Read the model definition and answer for the solid it produces. Units are mm, in the model's axes. A direction names the side the tool comes from. Give positions to 0.01 mm unless a question says otherwise; leave off trailing zeros. Write each loop counter-clockwise with the first axis right and the second up, starting at its lowest first coordinate (ties: lowest second). Pieces come first, ordered by that corner, then holes. Notation, with made-up numbers: (82, 44) -> (98, 44) arc R21 ccw to (98, 63) -> close; hole circle Ø7 at (10.5, 58). An arc over 180 degrees is marked (long way). Use a Markdown table: item, result.
from build123d import *

# Parameters (mm, degrees)
SKETCH1_W               = 325
SKETCH1_H               = 80
BOSS_EXTRUDE1_DEPTH     = 5
BOSS_EXTRUDE2_DEPTH     = 105
SKETCH3_R               = 4.5
CUT_EXTRUDE1_DEPTH      = 1
CUT_EXTRUDE1_DEPTH_BACK = 81
SKETCH4_W               = 120
SKETCH4_H               = 70
CUT_EXTRUDE2_DEPTH      = 105
SKETCH5_W               = 20
SKETCH5_H               = 20
CUT_EXTRUDE3_DEPTH      = 105


with BuildPart() as part:
    # Sketch1 → Boss-Extrude1 (new body)
    with BuildSketch(Plane(origin=(0, 0, 0), x_dir=(1, 0, 0), z_dir=(0, 1, 0))):
        with Locations((0, 45.507641921)):
            Rectangle(SKETCH1_W, SKETCH1_H)
    extrude(amount=-BOSS_EXTRUDE1_DEPTH)

    # Sketch2 → Boss-Extrude2 (add)
    with BuildSketch(Plane(origin=(0, 0, 0), x_dir=(1, 0, 0), z_dir=(0, 1, 0))):
        Polygon((-150.609375415, 80.507641921), (-162.5, 80.507641921), (-162.5, 85.507641921), (162.5, 85.507641921), (162.5, 5.507641921), (-162.5, 5.507641921), (-162.5, 10.507641921), (-150.609375415, 10.507641921), (153.5, 10.507641921), (153.5, 80.507641921), align=None)
    extrude(amount=BOSS_EXTRUDE2_DEPTH)

    # Sketch3 → Cut-Extrude1 (cut, two sides)
    with BuildSketch(Plane.XY.offset(-5.507641921)) as cut_extrude1_sk:
        with Locations((0, 50)):
            Circle(SKETCH3_R)
    extrude(amount=CUT_EXTRUDE1_DEPTH, mode=Mode.SUBTRACT)
    extrude(cut_extrude1_sk.sketch, amount=-CUT_EXTRUDE1_DEPTH_BACK, mode=Mode.SUBTRACT)

    # Sketch4 → Cut-Extrude2 (cut)
    with BuildSketch(Plane(origin=(0, 0, 0), x_dir=(1, 0, 0), z_dir=(0, 1, 0))):
        with Locations((-7.5, 45.507641921)):
            Rectangle(SKETCH4_W, SKETCH4_H)
    extrude(amount=-CUT_EXTRUDE2_DEPTH, mode=Mode.SUBTRACT)

    # Sketch5 → Cut-Extrude3 (cut)
    with BuildSketch(Plane(origin=(162.5, 0, 0), x_dir=(0, 0, -1), z_dir=(1, 0, 0))):
        Polygon((80.507641921, 105), (10.507641921, 105), (10.507641921, 60), (35.507641921, 60), (55.507641921, 60), (80.507641921, 60), align=None)
        with Locations((45.507641921, 50)):
            Rectangle(SKETCH5_W, SKETCH5_H)
        with BuildLine():
            Line((55.507641921, 40), (35.507641921, 40))
            ThreePointArc((35.507641921, 40), (45.507641921, 30), (55.507641921, 40))
        make_face()
    extrude(amount=-CUT_EXTRUDE3_DEPTH, mode=Mode.SUBTRACT)


solid = part.part
Item 1: A cutting plane is placed at A-A (z = -69.5). Give the vertices of the cut face in (x, y).
Return value:
| item | result |
|---|---|
| outline | (-162.5, -5) -> (-67.5, -5) -> (-67.5, 0) -> (-162.5, 0) -> close; (52.5, -5) -> (162.5, -5) -> (162.5, 60) -> (153.5, 60) -> (153.5, 0) -> (52.5, 0) -> close |
Item 2: For a pull along Z with two mould halves and no side action, classify faces 1 (the face through (153.5, 29.6, -45)), 2 (the face through (-0.98, 45.61, -82.97)), 3 (the face through (2, 37, -10.508)), 4 (the face through (-2, 37, -85.508)) as +Z half, -Z half, draft (parallel to the pull), parting line (faces both ways), or undercut.
Return value:
| item | result |
|---|---|
| face 1 | undercut |
| face 2 | draft |
| face 3 | undercut |
| face 4 | -Z half |
Item 3: A cutting plane is placed at C-C (x = 0). Give the vertices of the cut face in (y, z), then the cut area to 3 significant figures.
Return value:
| item | result |
|---|---|
| outline | (-5, -85.51) -> (45.5, -85.51) -> (45.5, -80.51) -> (-5, -80.51) -> close; (-5, -10.51) -> (45.5, -10.51) -> (45.5, -5.51) -> (-5, -5.51) -> close; (54.5, -85.51) -> (105, -85.51) -> (105, -80.51) -> (54.5, -80.51) -> close; (54.5, -10.51) -> (105, -10.51) -> (105, -5.51) -> (54.5, -5.51) -> close |
| area | 1,010 mm^2 |
Item 4: Each of these flat-tipped pins is pushed along its axis until it touches: P1, Ø7, axis at x = 0, y = 50, coming from the +Z side; P2, Ø7, axis at x = 158, z = -66, coming from the +Y side; P3, Ø10, axis at x = 123.5, z = -46, coming from the +Y side; P4, Ø3, axis at y = 53, z = -60.5, coming from the -X side. Where does it stop, or does it pass through?
Return value:
| item | result |
|---|---|
| P1 | through |
| P2 | y = 60 |
| P3 | y = 0 |
| P4 | x = 153.5 |
Item 5: A cutting plane is placed at B-B (y = 50). Give the vertices of the cut face in (x, z).
Return value:
| item | result |
|---|---|
| outline | (-162.5, -85.51) -> (-4.5, -85.51) -> (-4.5, -80.51) -> (-162.5, -80.51) -> close; (-162.5, -10.51) -> (-4.5, -10.51) -> (-4.5, -5.51) -> (-162.5, -5.51) -> close; (4.5, -85.51) -> (162.5, -85.51) -> (162.5, -55.51) -> (153.5, -55.51) -> (153.5, -80.51) -> (4.5, -80.51) -> close; (4.5, -10.51) -> (153.5, -10.51) -> (153.5, -35.51) -> (162.5, -35.51) -> (162.5, -5.51) -> (4.5, -5.51) -> close |
Item 6: A tool of negligible diameter and unlimited length cuts with its end or side. For faces 5 (the face through (158, 60, -68)), 6 (the face through (-2, -5, -82)), 7 (the face through (-116, 0, -46)), from which of +Z, -Z, +X, -X, +Y, -Y can it reach the whole face along a straight path? Write none if from no direction.
Return value:
| item | result |
|---|---|
| face 5 | +X, -X, +Y |
| face 6 | +Z, -Z, +X, -X, -Y |
| face 7 | -X, +Y |
Item 7: Straight lines are drawn through the part: line 1 along Z through (x, y) = (71, 89); line 2 along Y through (x, z) = (0, -7); line 3 along Y through (x, z) = (-88, -70). For each, find the intervals that lie inside material, in ascending order. Write a range as [from, to].
Return value:
| item | result |
|---|---|
| line 1 | [-85.51, -80.51], [-10.51, -5.51] |
| line 2 | [-5, 45.5], [54.5, 105] |
| line 3 | [-5, 0] |
Item 8: A cutting plane is placed at D-D (x = 122). Give the vertices of the cut face in (y, z).
Return value:
| item | result |
|---|---|
| outline | (-5, -85.51) -> (105, -85.51) -> (105, -80.51) -> (0, -80.51) -> (0, -10.51) -> (105, -10.51) -> (105, -5.51) -> (-5, -5.51) -> close |
